Verification items for the finished model (mm, model axes). A direction names the side the tool comes from. Give positions to 0.01 mm unless a question says otherwise; leave off trailing zeros. Write each loop counter-clockwise with the first axis right and the second up, starting at its lowest first coordinate (ties: lowest second). Pieces come first, ordered by that corner, then holes. Notation, with made-up numbers: (8, 74.25) -> (28, 74.25) arc R27 ccw to (28, 93.25) -> close; hole circle Ø10 at (48.5, 66.5). An arc over 180 degrees is marked (long way). Answer as CSV lines item,"result".
Autodesk Inventor part; units mm, degrees
ref_plane "YZ Plane" through (0, 0, 0) normal (1, 0, 0) x (0, 1, 0)
ref_plane "XZ Plane" through (0, 0, 0) normal (0, 1, 0) x (-1, 0, 0)
ref_plane "XY Plane" through (0, 0, 0) normal (0, 0, 1) x (1, 0, 0)
sketch "Skizze1" plane through (0, 0, 0) normal (0, 1, 0) x (-1, 0, 0)
  line L0 (-30, 100) -> (30, 100)
  line L1 (30, 100) -> (30, -100)
  line L2 (30, -100) -> (-30, -100)
  line L3 (-30, -100) -> (-30, 100)
  line L4 (-30, 100) -> (30, -100) construction
  line L5 (30, 100) -> (-30, -100) construction
  line L6 (0, -140) -> (0, 140)
  line L7 (-42, 0) -> (42, 0)
  point P0 (0, 0)
  point P1 (0, 0)
  dimension "d0" = 60
  dimension "d1" = 200
extrude "Extrusion1" add sketch "Skizze1" along normal blind 2
sketch "Skizze3" plane through (30, 0, 100) normal (1, 0, 0) x (0, 0, -1)
  line L0 (200, 2) -> (0, 2)
  line L1 (200, 0) -> (0, 0)
  line L2 (63.8142, 2) -> (136.1858, 2)
  line L3 (136.1858, 2) -> (136.1858, 0)
  line L4 (136.1858, 0) -> (63.8142, 0)
  line L5 (63.8142, 0) -> (63.8142, 2)
  line L6 (100, -0.4) -> (100, 2.4)
  point P0 (100, 0)
extrude "Extrusion3" add sketch "Skizze3" along normal blind 40
sketch "Skizze2" plane through (0, 2, 0) normal (0, 1, 0) x (1, 0, 0)
  line L0 (0, 140) -> (0, -140)
  line L1 (90, 0) -> (-50, 0)
  circle A0 centre (-23, 89.5) radius 1.6
  circle A1 centre (23, 89.5) radius 1.6
  line L2 (30, 100) -> (-30, 100)
  circle A2 centre (-23, 25.5) radius 1.6
  circle A3 centre (23, 25.5) radius 1.6
  circle A4 centre (-23, -89.5) radius 1.6
  circle A5 centre (23, -89.5) radius 1.6
  circle A6 centre (-23, -25.5) radius 1.6
  circle A7 centre (23, -25.5) radius 1.6
  line L3 (25, 83.9) -> (25, 31.1)
  line L4 (-25, 31.1) -> (-25, 83.9)
  line L5 (-30, 100) -> (-30, -100)
  line L6 (30, -100) -> (30, 100)
  line L7 (-17.4, 96) -> (17.4, 96)
  line L8 (17.4, 96) -> (17.4, 83.9)
  line L9 (-17.4, 83.9) -> (-17.4, 96)
  line L10 (-25, 83.9) -> (-17.4, 83.9)
  line L11 (17.4, 83.9) -> (25, 83.9)
  line L12 (17.4, -96) -> (-17.4, -96)
  line L13 (25, 31.1) -> (17.4, 31.1)
  line L14 (-17.4, 31.1) -> (-25, 31.1)
  line L15 (-30, -100) -> (30, -100)
  line L16 (-17.4, -31.1) -> (-26, -31.1)
  line L17 (-26, -31.1) -> (-26, -83.9)
  line L18 (-26, -83.9) -> (-17.4, -83.9)
  line L19 (17.4, -31.1) -> (26, -31.1)
  line L20 (26, -31.1) -> (26, -83.9)
  line L21 (26, -83.9) -> (17.4, -83.9)
  line L22 (-17.4, 19.9) -> (-26, 19.9)
  line L23 (-26, 19.9) -> (-26, -19.9)
  line L24 (-26, -19.9) -> (-17.4, -19.9)
  line L25 (17.4, 19.9) -> (26, 19.9)
  line L26 (26, 19.9) -> (26, -19.9)
  line L27 (26, -19.9) -> (17.4, -19.9)
  line L28 (-17.4, 19.9) -> (-17.4, 31.1)
  line L29 (17.4, 31.1) -> (17.4, 19.9)
  line L30 (17.4, -19.9) -> (17.4, -31.1)
  line L31 (17.4, -83.9) -> (17.4, -96)
  line L32 (-17.4, -96) -> (-17.4, -83.9)
  line L33 (-17.4, -31.1) -> (-17.4, -19.9)
  circle A8 centre (60, 23) radius 1.6
  circle A9 centre (60, -23) radius 1.6
  line L34 (30, 32.1858) -> (54.4, 32.1858)
  line L35 (54.4, -32.1858) -> (30, -32.1858)
  line L36 (30, -32.1858) -> (30, 32.1858)
  line L37 (30, -36.1858) -> (70, -36.1858)
  line L38 (30, 36.1858) -> (70, 36.1858)
  line L39 (54.4, 17.4) -> (66, 17.4)
  line L40 (66, 17.4) -> (66, -17.4)
  line L41 (66, -17.4) -> (54.4, -17.4)
  line L42 (70, 36.1858) -> (70, -36.1858)
  line L43 (54.4, 32.1858) -> (66, 32.1858)
  line L44 (66, 32.1858) -> (66, 28.6)
  line L45 (66, 28.6) -> (54.4, 28.6)
  line L46 (54.4, -28.6) -> (66, -28.6)
  line L47 (66, -28.6) -> (66, -32.1858)
  line L48 (66, -32.1858) -> (54.4, -32.1858)
  line L49 (54.4, 28.6) -> (54.4, 17.4)
  line L50 (54.4, -17.4) -> (54.4, -28.6)
  point P0 (0, 0)
  dimension "d2" = 2
  dimension "d4" = 3.2
  dimension "d5" = 3.2
  dimension "d6" = 10.5
  dimension "d7" = 10.5
  dimension "d8" = 23
  dimension "d9" = 23
  dimension "d10" = 3.2
  dimension "d11" = 3.2
  dimension "d12" = 23
  dimension "d13" = 23
  dimension "d14" = 25.5
  dimension "d15" = 25.5
  dimension "d16" = 5
  dimension "d17" = 5
  dimension "d23" = 4
  dimension "d24" = 4
  dimension "d25" = 4
  dimension "d26" = 4
  dimension "d27" = 4
  dimension "d30" = 4
  dimension "d31" = 4
  dimension "d33" = 4
  dimension "d34" = 4
  dimension "d35" = 4
  dimension "d36" = 4
  dimension "d37" = 4
  dimension "d38" = 4
  dimension "d39" = 4
  dimension "d40" = 4
  dimension "d41" = 4
  dimension "d42" = 4
  dimension "d43" = 4
  dimension "d44" = 4
  dimension "d45" = 4
  dimension "d48" = 12.6
  dimension "d49" = 12.6
  dimension "d50" = 12.6
  dimension "d51" = 12.6
  dimension "d52" = 12.6
  dimension "d53" = 12.6
  dimension "d58" = 3.2
  dimension "d59" = 3.2
  dimension "d60" = 23
  dimension "d61" = 23
  dimension "d64" = 37
  dimension "d65" = 37
  dimension "d66" = 4
  dimension "d68" = 4
  dimension "d69" = 4
  dimension "d70" = 4
  dimension "d71" = 4
  dimension "d72" = 4
  dimension "d73" = 4
  dimension "d74" = 4
  dimension "d75" = 4
  dimension "d76" = 4
  dimension "d77" = 15.6
  dimension "d78" = 15.6
extrude "Extrusion2" cut sketch "Skizze2" against normal up to surface (2 mm away) contours A0 | A1 | A2 | A3 | A4 | A5 | A6 | A7 | A8 | A9
sketch "Skizze4" plane through (0, 0, 0) normal (0, -1, 0) x (1, 0, 0)
  circle A0 centre (-23, -89.5) radius 1.6
  circle A1 centre (60, -23) radius 1.6
  circle A2 centre (23, -25.5) radius 1.6
  circle A3 centre (-23, 89.5) radius 1.6
  circle A4 centre (23, 25.5) radius 1.6
  circle A5 centre (23, -89.5) radius 1.6
  circle A6 centre (60, 23) radius 1.6
  circle A7 centre (-23, -25.5) radius 1.6
  circle A8 centre (23, 89.5) radius 1.6
  circle A9 centre (-23, 25.5) radius 1.6
  line L0 (-30, -100) -> (-30, 100)
  line L1 (30, -100) -> (-30, -100)
  line L2 (30, -36.1858) -> (30, -100)
  line L3 (30, -36.1858) -> (70, -36.1858)
  line L4 (70, 36.1858) -> (70, -36.1858)
  line L5 (30, 36.1858) -> (70, 36.1858)
  line L6 (30, 100) -> (30, 36.1858)
  line L7 (-30, 100) -> (30, 100)
  point P0 (0, 0)
extrude "Extrusion4" add sketch "Skizze4" along normal blind 2
sketch "Skizze5" plane through (0, 2, 0) normal (0, 1, 0) x (1, 0, 0)
  line L0 (-11.4, 79.9) -> (11.4, 79.9)
  line L1 (11.4, -79.9) -> (-11.4, -79.9)
  line L2 (-11.4, -79.9) -> (-11.4, 79.9)
  circle A0 centre (-23, 25.5) radius 1.6
  circle A1 centre (23, 25.5) radius 1.6
  circle A2 centre (23, 89.5) radius 1.6
  circle A3 centre (-23, -89.5) radius 1.6
  line L3 (11.4, 13.9) -> (55, 13.9)
  line L4 (55, 13.9) -> (55, -13.9)
  line L5 (55, -13.9) -> (11.4, -13.9)
  line L6 (70, 36.1858) -> (70, -36.1858)
  circle A4 centre (23, -25.5) radius 1.6
  line L7 (11.4, 79.9) -> (11.4, 13.9)
  line L8 (11.4, -13.9) -> (11.4, -79.9)
  line L9 (30, 36.1858) -> (30, 100)
  line L10 (30, -100) -> (30, -36.1858)
  point P0 (0, 0)
  dimension "d81" = 10
  dimension "d83" = 8
  dimension "d84" = 8
  dimension "d85" = 15
  dimension "d86" = 10
  dimension "d87" = 10
  dimension "d88" = 18.6
  dimension "d89" = 18.6
extrude "Extrusion5" cut sketch "Skizze5" against normal up to surface (4 mm away) contours L0 L7 L3 L4 L5 L8 L1 L2
properties part number "_3D-Druck"
1) Section check C-C (y = 1.1). State how many separate pieces and enclosed holes the cut face has, and give its area (3 significant figures).
Reported:
separate pieces,"1"
enclosed holes,"11"
area,"9,960 mm²"
2) Depth check by flat-ended pin: pin 1 (3 mm diameter, centred on x = 23, z = -89.5, fed in from +Y); pin 2 (2 mm diameter, centred on y = 0, z = -67.5, fed in from +X); pin 3 (1 mm diameter, centred on x = 53, y = 1, fed in from +Z). Enter the tip coordinate at first touch or a pass-through.
Reported:
pin 1,"through"
pin 2,"x = 30"
pin 3,"z = 36.19"
3) Scan lines: line 1 along Z through (x, y) = (-23, -1.1); line 2 along Z through (x, y) = (23, -0.85); line 3 along X through (y, z) = (0.35, -89.5). Record each from-to range of solid material in increasing order.
Reported:
line 1,"-100 to -91.1, -87.9 to -27.1, -23.9 to 23.9, 27.1 to 87.9, 91.1 to 100"
line 2,"-100 to -91.1, -87.9 to -27.1, -23.9 to -13.9, 13.9 to 23.9, 27.1 to 87.9, 91.1 to 100"
line 3,"-30 to -24.6, -21.4 to 21.4, 24.6 to 30"
4) Draft check along X on faces 6 (the flat face through (30, 0, -68)), 7 (the flat face through (0, 0, -100)), 8 (the flat face through (0, 0, 79.9)). Enter one of: +X half, -X half, draft (parallel to the pull), parting line (faces both ways), or undercut.
Reported:
face 6,"+X half"
face 7,"draft"
face 8,"undercut"
5) Section check A-A (z = 5.5). Record the boundary of the cut face in (x, y).
Reported:
outline,"(-30, -2) -> (-11.4, -2) -> (-11.4, 2) -> (-30, 2) -> close; (55, -2) -> (70, -2) -> (70, 2) -> (55, 2) -> close"
6) Tool access check on faces 1 (the flat face through (50, 0, 36.186)), 2 (the flat face through (0, 0, 100)), 3 (the flat face through (70, 0, 1)), 4 (the flat face through (50, 0, -36.186)), 5 (the flat face through (11.4, 0, -47)). Record the directions out of +Z, -Z, +X, -X, +Y, -Y that give a thin tool (end or side, any length) a straight path to the whole face; none if there is none.
Reported:
face 1,"+Z, +X, +Y, -Y"
face 2,"+Z, +X, -X, +Y, -Y"
face 3,"+Z, -Z, +X, +Y, -Y"
face 4,"-Z, +X, +Y, -Y"
face 5,"+Y, -Y"
7) Section check B-B (x = 46.5). Record the boundary of the cut face in (y, z).
Reported:
outline,"(-2, -36.19) -> (2, -36.19) -> (2, -13.9) -> (-2, -13.9) -> close; (-2, 13.9) -> (2, 13.9) -> (2, 36.19) -> (-2, 36.19) -> close"
